```python
from build123d import *

# Parameters (mm, degrees)
SKETCH1_R           = 4.75
BOSS_EXTRUDE1_DEPTH = 11


with BuildPart() as part:
    # Sketch1 → Boss-Extrude1 (new body)
    with BuildSketch(Plane(origin=(0, 0, 0), x_dir=(1, 0, 0), z_dir=(0, 1, 0))):
        with BuildLine():
            Line((0, 9), (88, 9))
            ThreePointArc((88, 9), (90.828427125, 7.828427125), (92, 5))
            Line((92, 5), (92, -4.118760913))
            ThreePointArc((92, -4.118760913), (88.083284346, -9), (82.46940199, -6.233868869))
            ThreePointArc((82.46940199, -6.233868869), (81.050506295, -4.43524348), (78.978362433, -3.458238822))
            Line((78.978362433, -3.458238822), (56.478362433, 1.324283815))
            ThreePointArc((56.478362433, 1.324283815), (51.57997572, -0.38691893), (50.837146839, -5.522151396))
            ThreePointArc((50.837146839, -5.522151396), (50.621338834, -7.879380022), (48.53631827, -9))
            Line((48.53631827, -9), (0, -9))
            ThreePointArc((0, -9), (-9, 0), (0, 9))
        make_face()
        Circle(SKETCH1_R, mode=Mode.SUBTRACT)
    extrude(amount=BOSS_EXTRUDE1_DEPTH)


solid = part.part
```
Can you work these out from the model? Positions are in its coordinate system, mm. A direction names the side the tool comes from. Give positions to 0.01 mm unless a question says otherwise; leave off trailing zeros. Write each loop counter-clockwise with the first axis right and the second up, starting at its lowest first coordinate (ties: lowest second). Pieces come first, ordered by that corner, then holes. Notation, with made-up numbers: (-5, 42.25) -> (33, 42.25) arc R25 ccw to (33, 55.25) -> close; hole circle Ø2 at (-23.75, -38). An arc over 180 degrees is marked (long way). One line per item, written item: value.
Q1. Imagine slicing it at B-B on y = 8.5. Please give me the cut outline in (x, z).
Results found:
outline: (0, -9) -> (88, -9) arc R4 ccw to (92, -5) -> (92, 4.12) arc R5 ccw to (82.47, 6.23) arc R5 cw to (78.98, 3.46) -> (56.48, -1.32) arc R5 cw to (50.84, 5.52) arc R2.5 ccw to (48.54, 9) -> (0, 9) arc R9 ccw to start; hole circle Ø9.5 at (0, 0)
Q2. Imagine slicing it at A-A on z = 0. Please give me the cut outline in (x, y), and give its area (3 significant figures).
Results found:
outline: (-9, 0) -> (-4.75, 0) -> (-4.75, 11) -> (-9, 11) -> close; (4.75, 0) -> (51.93, 0) -> (51.93, 11) -> (4.75, 11) -> close; (62.71, 0) -> (92, 0) -> (92, 11) -> (62.71, 11) -> close
area: 888 mm^2
Q3. Please list where these lines run through material, in increasing order: line 1 (Z direction, x = 10.5, y = 1); line 2 (X direction, y = 0.75, z = -3.25); line 3 (X direction, y = 7.75, z = -2.5). Write a range as [from, to].
Results found:
line 1: z = [-9, 9]
line 2: x = [-8.39, -3.46], [3.46, 92]
line 3: x = [-8.65, -4.04], [4.04, 92]
Q4. Which directions (+Z, -Z, +X, -X, +Y, -Y) give clear straight access to the entire face, cutting with the end or side of a thin tool? Please do faces 1 (the face through (42, 11, 0)), 2 (the face through (25, 5, 9)), 3 (the face through (50.64, 5.42, 7.85)), 4 (the face through (43, 5, -9)), 5 (the face through (67.89, 5.42, 1.1)).
Results found:
face 1: +Z, -Z, +X, -X, +Y
face 2: +Z, -X, +Y, -Y
face 3: +Y, -Y
face 4: -Z, +X, -X, +Y, -Y
face 5: +Z, +Y, -Y
Q5. We'd pull the mould along X, two halves only. Please class faces 6 (the face through (-9, 5, 0)), 7 (the face through (42, 0, 0)), 8 (the face through (90.797, 5.423, -7.859)), 9 (the face through (2.192, 5.423, 4.214)): +X half, -X half, draft (parallel to the pull), parting line (faces both ways), or undercut.
Results found:
face 6: -X half
face 7: draft
face 8: +X half
face 9: undercut
Q6. For P1, Ø2, axis at x = 57, y = 2, coming from the +Z side; P2, Ø2, axis at y = 2, z = -2.5, coming from the -X side; P3, Ø5.5, axis at x = 20, y = 3, coming from the +Z side, each with a flat end and sliding along its axis, tell me the tip position at first contact or that it passes through.
Results found:
P1: stops at z = -1
P2: stops at x = -8.87
P3: stops at z = 9
Q7. Imagine slicing it at C-C on x = 80. Please give me the cut outline in (y, z), and give its area (3 significant figures).
Results found:
outline: (0, -9) -> (11, -9) -> (11, 3.79) -> (0, 3.79) -> close
area: 141 mm^2
